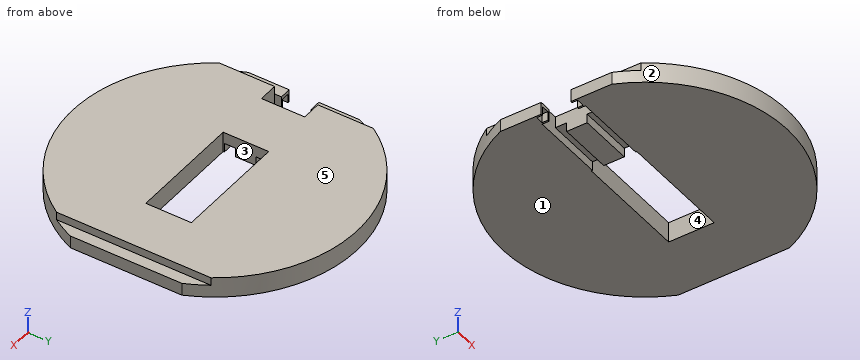
Solid Edge part; units mm, degrees
sketch "Sketch1" plane through (0, 0, 0) normal (0, 0, 1) x (1, 0, 0)
  circle A0 centre (0, 0) radius 125
extrude "Protrusion1" add sketch "Sketch1" along normal blind 18
sketch "Sketch2" plane through (0, 0, 18) normal (0, 0, 1) x (1, 0, 0)
  line L0 (115, 48.9898) -> (115, -48.9898)
  line L1 (149.5041, -48.9898) -> (115, -48.9898)
  line L2 (149.5041, 48.9898) -> (149.5041, -48.9898)
  line L3 (115, 48.9898) -> (149.5041, 48.9898)
extrude "ExtrudedCutout_1" cut sketch "Sketch2" against normal blind 18
sketch "Sketch3" plane through (-5, 0, 18) normal (0, 0, 1) x (0, 1, 0)
  line L0 (67.8233, -136.7696) -> (67.8233, -110)
  line L1 (67.8233, -110) -> (-67.8233, -110)
  line L2 (-67.8233, -110) -> (-67.8233, -136.7696)
  line L3 (-67.8233, -136.7696) -> (67.8233, -136.7696)
extrude "ExtrudedCutout_2" cut sketch "Sketch3" against normal blind 7
mirror "Mirror1" about plane through (0, 0, 0) normal (1, 0, 0) of "ExtrudedCutout_1", "ExtrudedCutout_2"
sketch "Sketch4" plane through (0, 0, 0) normal (0, 0, -1) x (-1, 0, 0)
  line L0 (115, 13) -> (105, 13)
  line L1 (105, 13) -> (105, 19)
  line L2 (105, 19) -> (88, 19)
  line L3 (88, 19) -> (88, -19)
  line L4 (88, -19) -> (105, -19)
  line L5 (105, -19) -> (105, -13)
  line L6 (105, -13) -> (115, -13)
  line L7 (115, -13) -> (115, 13)
  dimension "D1" = 88
  dimension "D2" = 105
extrude "ExtrudedCutout_6" cut sketch "Sketch4" against normal blind 18
sketch "Sketch5" plane through (0, 0, 0) normal (0, 0, -1) x (0, -1, 0)
  line L0 (-19, 88) -> (-19, -12)
  line L1 (-19, -12) -> (-9, -12)
  line L2 (-9, -12) -> (-9, 88)
  line L3 (-9, 88) -> (-19, 88)
  line L4 (19, 88) -> (19, -12)
  line L5 (19, -12) -> (9, -12)
  line L6 (9, -12) -> (9, 88)
  line L7 (9, 88) -> (19, 88)
extrude "ExtrudedCutout_7" cut sketch "Sketch5" against normal blind 8
sketch "Sketch6" plane through (0, 0, 0) normal (0, 0, -1) x (0, -1, 0)
  line L0 (-13, 113.5) -> (-18, 113.5)
  line L1 (-18, 113.5) -> (-18, 106.5)
  line L2 (-18, 106.5) -> (-13, 106.5)
  line L3 (-13, 106.5) -> (-13, 113.5)
  line L4 (13, 113.5) -> (18, 113.5)
  line L5 (18, 113.5) -> (18, 106.5)
  line L6 (18, 106.5) -> (13, 106.5)
  line L7 (13, 106.5) -> (13, 113.5)
  dimension "D1" = 13
  dimension "D2" = 13
extrude "ExtrudedCutout_8" cut sketch "Sketch6" against normal blind 8
sketch "Sketch7" plane through (0, 0, 0) normal (0, 0, -1) x (-1, 0, 0)
  line L0 (0, 20) -> (40, 20)
  line L1 (40, 20) -> (40, -20)
  line L2 (40, -20) -> (-60, -20)
  line L3 (-60, -20) -> (-60, 20)
  line L4 (-60, 20) -> (0, 20)
extrude "ExtrudedCutout_9" cut sketch "Sketch7" against normal blind 18
properties material "Wood, Ash"
Source: CAD feature listing. Evaluate the final solid. Frame: model axes, mm. Face numbers are marked on the shaded views. A direction names the side the tool comes from. Coordinates: 2 decimals unless noted, no trailing zeros. Order: outer loops, then holes, each group sorted by start corner. A loop starts at its lowest first (then second) coordinate and runs counter-clockwise, first axis right, second up.
Item 1: Set-up query: the marked faces 4 and 5. Return all of +Z, -Z, +X, -X, +Y, -Y with unobstructed straight access to the full face (end or side cutting, diameter ignored); none if empty.
Output values:
face 4: +Z, -Z
face 5: +Z, +X, -X, +Y, -Y
Item 2: Cut plane D-D (x = -48). Return loops of the section in (y, z).
Output values:
outline: (-115.42, 0) - (-19, 0) - (-19, 8) - (-9, 8) - (-9, 0) - (9, 0) - (9, 8) - (19, 8) - (19, 0) - (115.42, 0) - (115.42, 18) - (-115.42, 18) - close
Item 3: Cut plane C-C (x = 56). Return loops of the section in (y, z), plus the area to 3 significant figures.
Output values:
outline: (-111.75, 0) - (-20, 0) - (-20, 18) - (-111.75, 18) - close; (20, 0) - (111.75, 0) - (111.75, 18) - (20, 18) - close
area: 3,300 mm2
Item 4: Cut plane B-B (z = 4). Return loops of the section in (x, y).
Output values:
outline: (-115, -48.99) arc R125 ccw to (115, -48.99) - (115, 48.99) arc R125 ccw to (-115, 48.99) - (-115, 13) - (-113.5, 13) - (-113.5, 18) - (-106.5, 18) - (-106.5, 13) - (-105, 13) - (-105, 19) - (-40, 19) - (-40, 20) - (60, 20) - (60, -20) - (-40, -20) - (-40, -19) - (-105, -19) - (-105, -13) - (-106.5, -13) - (-106.5, -18) - (-113.5, -18) - (-113.5, -13) - (-115, -13) - close; (-88, -9) - (-40, -9) - (-40, 9) - (-88, 9) - close
Item 5: Material intervals for line 1 (X direction, y = -42, z = 17); line 2 (Y direction, x = -0.5, z = 9); line 3 (Y direction, x = -21.5, z = 4.5), sorted ascending.
Output values:
line 1: x = -105 to 105
line 2: y = -125 to -20, 20 to 125
line 3: y = -123.14 to -20, 20 to 123.14
Item 6: Cut plane A-A (y = 5.5). Return loops of the section in (x, z).
Output values:
outline: (-88, 0) - (-40, 0) - (-40, 18) - (-88, 18) - close; (60, 0) - (115, 0) - (115, 11) - (105, 11) - (105, 18) - (60, 18) - close
Item 7: First-contact query: P1, Ø2, axis at x = -110.5, z = 5.5, coming from the +Y side; P2, Ø7.5, axis at x = -109, z = 5.5, coming from the -Y side; P3, Ø5, axis at x = -54, y = 12.5, coming from the -Z side; P4, Ø12, axis at x = 59.5, y = 17.5, coming from the -Z side. Flat tips, straight axial feed; report the tip coordinate or a pass-through.
Output values:
P1: stops at y = 60.29
P2: stops at y = -67.43
P3: stops at z = 8
P4: stops at z = 0
Item 8: Pull-direction query (Y, two-part tool) for the marked faces 1, 2 and 3; classes: pulls with the +Y half, pulls with the -Y half, needs draft (parallel to the pull), parting line crosses it, or undercut.
Output values:
face 1: needs draft
face 2: pulls with the -Y half
face 3: undercut
